```python
from build123d import *

# Parameters (mm, degrees)
BOSS_EXTRU_4_DEPTH        = 1
BOSS_EXTRU_5_DEPTH        = 198
COQUE2_T                  = -2
BOSS_EXTRU_6_DEPTH        = 2
ENL_V_START               = -2
ENL_V_MAT_EXTRU_3_DEPTH   = 2
ESQUISSE18_W              = 1
ESQUISSE18_H              = 196
BOSS_EXTRU_7_DEPTH        = 20
SYM_TRIE3_COPY_1_SKETCH_W = 1
SYM_TRIE3_COPY_1_SKETCH_H = 196
SYM_TRIE3_COPY_1_DEPTH    = 20
ESQUISSE19_W              = 2
ESQUISSE19_H              = 196
BOSS_EXTRU_8_DEPTH        = 20
SYM_TRIE5_COPY_1_SKETCH_W = 2
SYM_TRIE5_COPY_1_SKETCH_H = 196
SYM_TRIE5_COPY_1_DEPTH    = 20


with BuildPart() as part:
    # Esquisse1 → Boss.-Extru.4 (new body)
    with BuildSketch(Plane(origin=(0, 0, 0), x_dir=(1, 0, 0), z_dir=(0, 1, 0))):
        with BuildLine():
            Line((-280, 200), (280, 200))
            ThreePointArc((280, 200), (294.142135624, 194.142135624), (300, 180))
            Line((300, 180), (300, -180))
            ThreePointArc((300, -180), (294.142135624, -194.142135624), (280, -200))
            Line((280, -200), (-280, -200))
            ThreePointArc((-280, -200), (-294.142135624, -194.142135624), (-300, -180))
            Line((-300, -180), (-300, 180))
            ThreePointArc((-300, 180), (-294.142135624, 194.142135624), (-280, 200))
        make_face()
    boss_extru_4 = extrude(amount=BOSS_EXTRU_4_DEPTH)

    # Esquisse3 → Boss.-Extru.5 (add)
    with BuildSketch(Plane(origin=(0, 1, 0), x_dir=(1, 0, 0), z_dir=(0, 1, 0))):
        with BuildLine():
            Line((-260, 180), (260, 180))
            ThreePointArc((260, 180), (274.142135624, 174.142135624), (280, 160))
            Line((280, 160), (280, -160))
            ThreePointArc((280, -160), (274.142135624, -174.142135624), (260, -180))
            Line((260, -180), (-260, -180))
            ThreePointArc((-260, -180), (-274.142135624, -174.142135624), (-280, -160))
            Line((-280, -160), (-280, 160))
            ThreePointArc((-280, 160), (-274.142135624, 174.142135624), (-260, 180))
        make_face()
    extrude(amount=BOSS_EXTRU_5_DEPTH)

    # Coque2
    coque2_openings = [part.faces().sort_by_distance(p)[0] for p in [
        (0, 199, 0),
    ]]
    offset(amount=COQUE2_T, openings=coque2_openings, kind=Kind.INTERSECTION)



with BuildPart() as body_2:
    # Esquisse12 → Boss.-Extru.6 (new body)
    with BuildSketch(Plane(origin=(0, 197, 0), x_dir=(1, 0, 0), z_dir=(0, 1, 0))):
        with BuildLine():
            Line((-280, 200), (280, 200))
            ThreePointArc((280, 200), (294.142135624, 194.142135624), (300, 180))
            Line((300, 180), (300, -180))
            ThreePointArc((300, -180), (294.142135624, -194.142135624), (280, -200))
            Line((280, -200), (-280, -200))
            ThreePointArc((-280, -200), (-294.142135624, -194.142135624), (-300, -180))
            Line((-300, -180), (-300, 180))
            ThreePointArc((-300, 180), (-294.142135624, 194.142135624), (-280, 200))
        make_face()
    extrude(amount=BOSS_EXTRU_6_DEPTH)

    # Esquisse17 → Enlèv. mat.-Extru.3 (cut)
    with BuildSketch(Plane(origin=(0, 199, 0), x_dir=(1, 0, 0), z_dir=(0, 1, 0)).offset(ENL_V_START)):
        with BuildLine():
            Line((-260, 180), (260, 180))
            ThreePointArc((260, 180), (274.142135624, 174.142135624), (280, 160))
            Line((280, 160), (280, -160))
            ThreePointArc((280, -160), (274.142135624, -174.142135624), (260, -180))
            Line((260, -180), (-260, -180))
            ThreePointArc((-260, -180), (-274.142135624, -174.142135624), (-280, -160))
            Line((-280, -160), (-280, 160))
            ThreePointArc((-280, 160), (-274.142135624, 174.142135624), (-260, 180))
        make_face()
    extrude(amount=ENL_V_MAT_EXTRU_3_DEPTH, mode=Mode.SUBTRACT)


with BuildPart() as part_1:
    add(part.part)

    add(body_2.part)  # Boss.-Extru.7 merges body 2
    # Esquisse18 → Boss.-Extru.7 (add)
    with BuildSketch(Plane(origin=(280, 0, 0), x_dir=(0, 0, -1), z_dir=(1, 0, 0))):
        with Locations((-159.5, 99)):
            Rectangle(ESQUISSE18_W, ESQUISSE18_H)
    boss_extru_7 = extrude(amount=BOSS_EXTRU_7_DEPTH)


with BuildPart() as sym_trie1_1:
    # Symétrie1: Boss.-Extru.4 across plane
    add(boss_extru_4.mirror(Plane.XY))


with BuildPart() as part_2:
    add(part_1.part)

    # Symétrie1 united with what the copies to: union Symétrie1_1
    add(sym_trie1_1.part)

    # Symétrie2: Boss.-Extru.7 across plane
    add(boss_extru_7.mirror(Plane.XY))

    # Symétrie3: Boss.-Extru.7 across plane
    add(boss_extru_7.mirror(Plane(origin=(0, 0, 0), x_dir=(0, 0, 1), z_dir=(1, 0, 0))))

    # Symétrie3 copy 1 sketch → Symétrie3 copy 1 (add)
    with BuildSketch(Plane.ZY.offset(280)):
        with Locations((-159.5, 99)):
            Rectangle(SYM_TRIE3_COPY_1_SKETCH_W, SYM_TRIE3_COPY_1_SKETCH_H)
    extrude(amount=SYM_TRIE3_COPY_1_DEPTH)

    # Esquisse19 → Boss.-Extru.8 (add)
    with BuildSketch(Plane.XY.offset(180)):
        with Locations((-259, 99)):
            Rectangle(ESQUISSE19_W, ESQUISSE19_H)
    boss_extru_8 = extrude(amount=BOSS_EXTRU_8_DEPTH)

    # Symétrie4: Boss.-Extru.8 across plane
    add(boss_extru_8.mirror(Plane(origin=(0, 0, 0), x_dir=(0, 0, 1), z_dir=(1, 0, 0))))

    # Symétrie5: Boss.-Extru.8 across plane
    add(boss_extru_8.mirror(Plane.XY))

    # Symétrie5 copy 1 sketch → Symétrie5 copy 1 (add)
    with BuildSketch(Plane(origin=(0, 0, -180), x_dir=(-1, 0, 0), z_dir=(0, 0, -1))):
        with Locations((-259, 99)):
            Rectangle(SYM_TRIE5_COPY_1_SKETCH_W, SYM_TRIE5_COPY_1_SKETCH_H)
    extrude(amount=SYM_TRIE5_COPY_1_DEPTH)


solid = part_2.part
```
Can you work these out from the model? Positions are in its coordinate system, mm. A direction names the side the tool comes from. Coordinates: 2 decimals unless noted, no trailing zeros. Loops run counter-clockwise (first coordinate to the right, second up) from the corner with the lowest first, then second, coordinate; pieces in that order, holes last.
1) Imagine slicing it at B-B on x = 30. List the corners of the cut face in (y, z) for me.
2) Which directions (+Z, -Z, +X, -X, +Y, -Y) give clear straight access to the entire face, cutting with the end or side of a thin tool? Please do faces 1 (the flat face through (280, 197, 180)), 2 (the flat face through (-278, 99, 2)), 3 (the flat face through (-4, 98, -180)), 4 (the flat face through (-290, 1, -2)), 5 (the cylindrical face through (-273.986, 97.628, 174.297)).
3) I need wall thicknesses on probe 1 along Z at (x, y) = (13.5, 108); probe 2 along X at (y, z) = (125.5, -98); probe 3 along X at (y, z) = (101, -184). Which ranges of each line are inside material? Lowest first, please.
4) For pin 1 (1.5 mm diameter, centred on x = -209, z = 14.5, fed in from +Y); pin 2 (16 mm diameter, centred on x = -290.5, y = 71, fed in from -Z); pin 3 (10 mm diameter, centred on x = -289.5, y = 70, fed in from +Z); pin 4 (2 mm diameter, centred on x = 21, z = 118, fed in from -Y), each with a flat end and sliding along its axis, tell me the tip position at first contact or that it passes through.
5) Thinking about a two-plate mould opening in Y: for faces 6 (the flat face through (4, 2, -2)), 7 (the cylindrical face through (293.986, 0.493, -194.297)), 8 (the flat face through (-280, 1, -180)), which applies, pulls with the +Y half, pulls with the -Y half, needs draft (parallel to the pull), parting line crosses it, or undercut?
6) Imagine slicing it at A-A on z = -37. List the corners of the cut face in (x, y) for me, plus the area to 3 significant figures.
Completed:
1. outline: (0, -200) - (1, -200) - (1, -180) - (197, -180) - (197, -200) - (199, -200) - (199, -178) - (2, -178) - (2, 178) - (199, 178) - (199, 200) - (197, 200) - (197, 180) - (1, 180) - (1, 200) - (0, 200) - close
2. face 1: +Z, +X
2. face 2: +Y
2. face 3: -Z
2. face 4: -X
2. face 5: +Z, -X
3. probe 1: z = -180 to -178, 178 to 180
3. probe 2: x = -280 to -278, 278 to 280
3. probe 3: x = -260 to -258, 258 to 260
4. pin 1: stops at y = 2
4. pin 2: stops at z = -160
4. pin 3: stops at z = 160
4. pin 4: stops at y = 0
5. face 6: pulls with the +Y half
5. face 7: needs draft
5. face 8: undercut
6. outline: (-300, 0) - (300, 0) - (300, 1) - (280, 1) - (280, 197) - (300, 197) - (300, 199) - (278, 199) - (278, 2) - (-278, 2) - (-278, 199) - (-300, 199) - (-300, 197) - (-280, 197) - (-280, 1) - (-300, 1) - close
6. area: 2,030 mm2
